Part model, mm, in its own coordinate system. Face numbers are marked on the shaded views. Round coordinates to 2 decimals unless told otherwise and drop trailing zeros. Loops run counter-clockwise (first coordinate to the right, second up) from the corner with the lowest first, then second, coordinate; pieces in that order, holes last. Notation, with made-up numbers: M 77.25,20 L 89.25,20 A26 ccw 89.25,59 Z; hole C 2.5,5 d6. An arc over 180 degrees is marked long. Write each question's results on one line, items separated by ' | '.
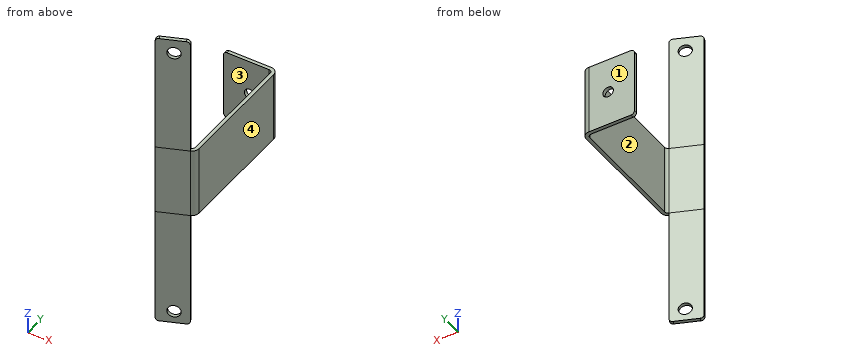
Autodesk Inventor part; units mm, degrees
ref_plane "YZ Plane" through (0, 0, 0) normal (1, 0, 0) x (0, 1, 0)
ref_plane "XZ Plane" through (0, 0, 0) normal (0, 1, 0) x (-1, 0, 0)
ref_plane "XY Plane" through (0, 0, 0) normal (0, 0, 1) x (1, 0, 0)
sketch "Sketch1" plane through (0, 0, 0) normal (0, 1, 0) x (-1, 0, 0)
  line L0 (0, 20) -> (-30, 20)
  line L1 (-30, 20) -> (-30, -20)
  line L2 (-30, -20) -> (0, -20)
  line L3 (0, -20) -> (0, 20)
  point P0 (0, 0)
  dimension "d0" = 20
  dimension "d1" = 20
  dimension "d2" = 0
  dimension "d3" = 30
extrude "Plate1" add sketch "Sketch1" along normal blind 2
sketch "Sketch2" plane through (28, 2, -20) normal (1, 0, 0) x (0, -1, 0)
  line L0 (0, 40) -> (0, 0)
  line L1 (0, 0) -> (74, 0)
  line L2 (74, 0) -> (74, 40)
  line L3 (74, 40) -> (0, 40)
edge flange "Flange1" height 74 angle -90 thickness 2 bend radius 2 thickness toward (1, 0, 0) relief tear relief width 2 relief depth 1 edges at (30, 2, 0) wall of the first edge with corners at (28, 2, 20) (28, 2, -20) (28, -72, -20) (28, -72, 20)
bend "Bend1"
corner "Corner1"
sketch "Sketch3" plane through (29.2508, -70.1456, 20) normal (0.3746066, -0.9271839, 0) x (0.9271839, 0.3746066, 0)
  line L0 (0, -40) -> (0, 0)
  line L1 (0, 0) -> (-20, 0)
  line L2 (-20, 0) -> (-20, -40)
  line L3 (-20, -40) -> (0, -40)
edge flange "Flange2" height 20 angle 68 thickness 2 bend radius 2 thickness toward (0.3746066, -0.9271839, 0) relief tear relief width 2 relief depth 1 edges at (28, -72, 0) wall of the first edge with corners at (29.2508, -70.1456, -20) (29.2508, -70.1456, 20) (10.7071, -77.6378, 20) (10.7071, -77.6378, -20)
bend "Bend2"
corner "Corner2"
sketch "Sketch4" plane through (11.4563, -79.4921, 20) normal (0.3746066, -0.9271839, 0) x (-0.9271839, -0.3746066, 0)
  line L0 (-17.302, 40) -> (-17.302, 0)
  line L1 (0, 0) -> (-17.302, 0)
  line L2 (0, 40) -> (0, 0)
  line L3 (-17.302, 40) -> (0, 40)
  line L4 (-17.302, -67.5) -> (0, -67.5)
  line L5 (0, -67.5) -> (0, 107.5)
  line L6 (0, 107.5) -> (-17.302, 107.5)
  line L7 (-17.302, 107.5) -> (-17.302, -67.5)
  point P0 (-19.1562, 20)
  dimension "d26" = 87.5
  dimension "d27" = 87.5
  dimension "d28" = 0
  dimension "d30" = 0
extrude "Extrusion1" add sketch "Sketch4" against normal blind 2 contours L7 L6 L5 L3 | L1 L5 L4 L7
sketch "Sketch5" plane through (0, 2, 0) normal (0, 1, 0) x (1, 0, 0)
  circle A0 centre (15, 0) radius 3
  line L0 (36, 0) -> (-6, 0)
  point P0 (0, 0)
  dimension "d51" = 6
  dimension "d52" = 0
  dimension "d53" = 15
extrude "Extrusion2" cut sketch "Sketch5" against normal blind 2
sketch "Sketch6" plane through (27.4984, -73.0107, 87.5) normal (0.3746066, -0.9271839, 0) x (-0.9271839, -0.3746066, 0)
  circle A0 centre (8, 8) radius 3.5
  line L0 (0, 107.5) -> (0, 67.5)
  line L1 (0, 67.5) -> (0, 0)
  line L2 (0, 0) -> (17.302, 0)
  line L3 (17.302, 0) -> (17.302, 175)
  line L4 (17.302, 175) -> (0, 175)
  line L5 (0, 175) -> (0, 107.5)
  circle A1 centre (8, 168) radius 3.5
  point P0 (-1.8542, 87.5)
  dimension "d38" = 7
  dimension "d39" = 8
  dimension "d40" = 8
  dimension "d43" = 160
extrude "Extrusion3" cut sketch "Sketch6" against normal blind 2 contours A0 | A1
fillet "Fillet1" radius 2 6 edges at (0, 1, 20) (0, 1, -20) (11.0817, -78.5649, 87.5) (27.1238, -72.0835, 87.5) (11.0817, -78.5649, -87.5) (27.1238, -72.0835, -87.5)
equation "\"d4\" = Thickness"
equation "\"d5\" = BendReliefWidth"
equation "\"d6\" = BendReliefDepth"
equation "\"d7\" = MinimumRemnant"
equation "\"d8\" = TransitionRadius"
equation "\"d11\" = BendRadius"
equation "\"d12\" = CornerReliefSize"
equation "\"d13\" = GapSize"
equation "\"d14\" = JacobiRadiusSize"
equation "\"d15\" = BendReliefWidth"
equation "\"d16\" = BendReliefDepth"
equation "\"d17\" = MinimumRemnant"
equation "\"d18\" = TransitionRadius"
equation "\"d21\" = BendRadius"
equation "\"d22\" = CornerReliefSize"
equation "\"d23\" = GapSize"
equation "\"d24\" = JacobiRadiusSize"
equation "\"BendRadius\" = Thickness"
equation "\"BendReliefWidth\" = Thickness"
equation "\"BendReliefDepth\" = 0.5 * Thickness"
equation "\"CornerReliefSize\" = 4 * Thickness"
equation "\"MinimumRemnant\" = 2 * Thickness"
equation "\"TransitionRadius\" = BendRadius"
equation "\"JacobiRadiusSize\" = BendRadius"
equation "\"GapSize\" = Thickness"
properties part number "Bottom Mount" material "Stainless Steel"
Item 1: Band-saw the part on B-B on x = 4. Give the cut face in (y, z), and give its area (3 significant figures).
Filled sheet:
outline: M 0,-20 L 2,-20 L 2,20 L 0,20 Z | area: 80.0 mm^2
Item 2: Two-plate mould, pull along Y, no slides. Class the marked faces 1, 2, 3 and 4: +Y half, -Y half, draft (parallel to the pull), parting line (faces both ways), or undercut.
Filled sheet:
face 1: +Y half | face 2: undercut | face 3: undercut | face 4: draft
Item 3: Drop flat-ended pins along their axis: P1, Ø8, axis at x = 22.5, y = -59, coming from the -Z side; P2, Ø5.5, axis at x = 15, z = 0, coming from the -Y side; P3, Ø6, axis at x = 27, y = -40, coming from the +Z side; P4, Ø6, axis at x = 18.5, z = -42, coming from the +Y side. Give the stop position or say it passes through.
Filled sheet:
P1: through | P2: y = -79.17 | P3: z = 20 | P4: y = -73.28
Item 4: Wall check: L1, parallel to Z at x = 15, y = 0.65; L2, parallel to X at y = -44.5, z = 10; L3, parallel to Y at x = 24.75, z = 17.5. Give the ranges that are in metal, low to high.
Filled sheet:
L1: -20 to -3, 3 to 20 | L2: 28 to 30 | L3: -74.12 to -71.96, 0 to 2
Item 5: Band-saw the part on A-A on z = 0. Give the cut face in (x, y), and give its area (3 significant figures).
Filled sheet:
outline: M 0,0 L 12,0 L 12,2 L 0,2 Z; M 10.71,-77.64 L 11.46,-79.49 L 27.5,-73.01 A4 ccw 30,-69.3 L 30,-2 A4 ccw 26,2 L 18,2 L 18,0 L 26,0 A2 cw 28,-2 L 28,-69.3 A2 cw 26.75,-71.16 Z | area: 226 mm^2
Item 6: Band-saw the part on C-C on z = 40. Give the cut face in (x, y).
Filled sheet:
outline: M 10.71,-77.64 L 11.46,-79.49 L 27.5,-73.01 L 26.75,-71.16 Z
